Input: part model. Units: mm. Frame: model coordinates. Give positions to 0.01 mm unless a question says otherwise; leave off trailing zeros. Loops run counter-clockwise (first coordinate to the right, second up) from the corner with the lowest first, then second, coordinate; pieces in that order, holes last. Notation, with made-up numbers: (-16, 9) - (40, 9) arc R24 ccw to (40, 30) - close; hole circle Ø8 at (35.25, 70.25). An arc over 180 degrees is marked (long way). Answer as a JSON object with one key per item and string values.
from build123d import *

# Parameters (mm, degrees)
SKETCH2_W               = 101.6
SKETCH2_H               = 50.8
BOSS_EXTRUDE1_DEPTH     = 122.512802726
BOSS_EXTRUDE2_DEPTH     = 50.8
CUT_EXTRUDE1_DEPTH      = 261.524644331
CUT_EXTRUDE1_DEPTH_BACK = 261.524644331
SKETCH4_W               = 12.7
SKETCH4_H               = 234.456585115


with BuildPart() as part:
    # Sketch2 → Boss-Extrude1 (new body)
    with BuildSketch(Plane.XY):
        with Locations((50.8, 25.4)):
            Rectangle(SKETCH2_W, SKETCH2_H)
    extrude(amount=BOSS_EXTRUDE1_DEPTH)

    # Sketch3 → Boss-Extrude2 (add)
    with BuildSketch(Plane(origin=(0, 50.8, 0), x_dir=(1, 0, 0), z_dir=(0, 1, 0))):
        Polygon((101.6, -122.512802726), (15.9196024, -234.456585115), (0, -234.456585115), (0, -122.512802726), align=None)
    extrude(amount=-BOSS_EXTRUDE2_DEPTH)

    # Sketch4 → Cut-Extrude1 (cut, two sides: drawn at the far end of the back side and taken through both)
    with BuildSketch(Plane(origin=(0, 50.8, 0), x_dir=(1, 0, 0), z_dir=(0, 1, 0)).offset(-CUT_EXTRUDE1_DEPTH_BACK)):
        with Locations((6.35, -117.228292558)):
            Rectangle(SKETCH4_W, SKETCH4_H)
    extrude(amount=CUT_EXTRUDE1_DEPTH + CUT_EXTRUDE1_DEPTH_BACK, mode=Mode.SUBTRACT)


solid = part.part
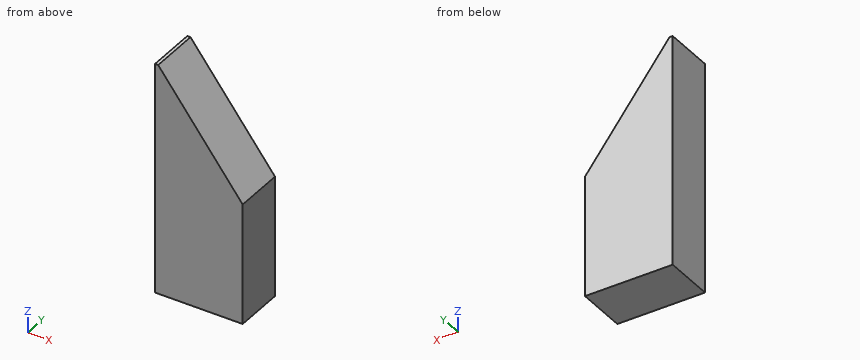
Item 1: Cut plane B-B (z = 214). Return loops of the section in (x, y), then the cut area to 3 significant figures.
Geometry check:
{"outline": "(12.7, 0) - (31.58, 0) - (31.58, 50.8) - (12.7, 50.8) - close", "area": "959 mm2"}
Item 2: Contact query for a flat-ended pin moving along its axis: P1, Ø10, axis at x = 58.5, y = 22.5, coming from the +Z side. Output: stop coordinate, or through.
Geometry check:
{"P1": "stops at z = 185.36"}
Item 3: Material intervals for line 1 (X direction, y = 19.5, z = 172); line 2 (X direction, y = 33.5, z = 214); line 3 (Z direction, x = 29, y = 40.5), sorted ascending. Write a range as [from, to].
Geometry check:
{"line 1": "x = [12.7, 63.72]", "line 2": "x = [12.7, 31.58]", "line 3": "z = [0, 217.37]"}
Item 4: Cut plane C-C (x = 27.5). Return loops of the section in (y, z).
Geometry check:
{"outline": "(0, 0) - (50.8, 0) - (50.8, 219.33) - (0, 219.33) - close"}
Item 5: Cut plane A-A (y = 35). Return loops of the section in (x, z).
Geometry check:
{"outline": "(12.7, 0) - (101.6, 0) - (101.6, 122.51) - (15.92, 234.46) - (12.7, 234.46) - close"}
